from build123d import *

# Parameters (mm, degrees)
F0_R     = 4.4
F1_DEPTH = 1


with BuildPart() as f1:
    # F0 (on Front) → F1 (new body)
    with BuildSketch(Plane.XZ):
        with BuildLine():
            ThreePointArc((-1.4986815922, 5.1042757445), (-10.8737353251, 1.8109915545), (-1, 2.9275505456))
            ThreePointArc((-1, 2.9275505456), (-1.0654410934, 3.733855945), (-1.2600513589, 4.5190551417))
            ThreePointArc((-1.2600513589, 4.5190551417), (-1.3701106972, 4.81543959), (-1.4986815922, 5.1042757445))
        make_face()
        with Locations((-6, 2.9275505456)):
            Circle(F0_R, mode=Mode.SUBTRACT)
        with BuildLine():
            ThreePointArc((-1.4986815922, 5.1042757445), (-1.3701106972, 4.81543959), (-1.2600513589, 4.5190551417))
            add(Edge.make_bspline(
                [(-1.2600513589, 4.5190551417), (-0.3321453987, 5.1084347069), (0.2222434123, 5.0197322853), (1.305815297, 4.6493606322)],
                knots=[0, 0, 0, 0, 2.5691732555, 2.5691732555, 2.5691732555, 2.5691732555], degree=3))
            ThreePointArc((1.305815297, 4.6493606322), (1.408443121, 4.9068447194), (1.525181814, 5.1582459982))
            add(Edge.make_bspline(
                [(-1.4986815922, 5.1042757445), (0, 5.9878164902), (1.4394625627, 5.1295237069), (1.525181814, 5.1582459982)],
                knots=[0, 0, 0, 0, 0.9403135209, 0.9403135209, 0.9403135209, 0.9403135209], degree=3))
        make_face()
        with BuildLine():
            ThreePointArc((1.525181814, 5.1582459982), (1.408443121, 4.9068447194), (1.305815297, 4.6493606322))
            ThreePointArc((1.305815297, 4.6493606322), (5.1256212248, -1.9954019991), (11, 2.9275505456))
            ThreePointArc((11, 2.9275505456), (10.9952473554, 3.1455043436), (10.9809984568, 3.3630437989))
            ThreePointArc((10.9809984568, 3.3630437989), (10.9614239437, 3.5474476752), (10.9350249024, 3.7309988718))
            ThreePointArc((10.9350249024, 3.7309988718), (6.7558272917, 7.8700929182), (1.5306314581, 5.1691448079))
            add(Edge.make_bspline(
                [(1.525181814, 5.1582459982), (1.5306228506, 5.160069148), (1.5306095387, 5.165466158), (1.5306314581, 5.1691448079)],
                knots=[0.9403135209, 0.9403135209, 0.9403135209, 0.9403135209, 1, 1, 1, 1], degree=3))
        make_face()
        with Locations((6, 2.9275505456)):
            Circle(F0_R, mode=Mode.SUBTRACT)
        with BuildLine():
            ThreePointArc((10.9350249024, 3.7309988718), (10.9614239437, 3.5474476752), (10.9809984568, 3.3630437989))
            Line((10.9809984568, 3.3630437989), (11.1943203956, 3.3630437989))
            Line((11.1943203956, 3.3630437989), (11.1943203956, -15.5131826177))
            Line((11.1943203956, -15.5131826177), (11.5463633525, -15.5131826177))
            Line((11.5463633525, -15.5131826177), (11.5463633525, 3.7309988718))
            Line((11.5463633525, 3.7309988718), (10.9350249024, 3.7309988718))
        make_face()
    extrude(amount=F1_DEPTH)


solid = f1.part
Could you check a few things on this model? Use its own coordinates, in mm. A direction names the side the tool comes from. Give positions to 0.01 mm unless a question says otherwise; leave off trailing zeros. Loops run counter-clockwise (first coordinate to the right, second up) from the corner with the lowest first, then second, coordinate; pieces in that order, holes last. Notation, with made-up numbers: M 0.5,-17.75 L 55.5,-17.75 A15 cw 55.5,-0.75 Z; hole C 71,76.25 d7. An arc over 180 degrees is marked long. Answer as a JSON object with one key per item and string values.
Q1. Suppose I cut it at D-D, the plane y = -0.8. State how many separate pieces and enclosed holes the cut face has, plus the area to 3 significant figures.
Values found:
{"separate pieces": "1", "enclosed holes": "2", "area": "44.0 mm²"}
Q2. If I drill on probe 1 along X at (y, z) = (-0.25, 3); probe 2 along Z at (x, y) = (-6, -0.25); probe 3 along X at (y, z) = (-0.55, 6.5), over which ranges is the centre line in solid material (lowest first)? Write a range as [from, to].
Values found:
{"probe 1": "x = [-11, -10.4], [-1.6, -1], [1, 1.6], [10.4, 11], [11.19, 11.55]", "probe 2": "z = [-2.07, -1.47], [7.33, 7.93]", "probe 3": "x = [-9.5, -8.57], [-3.43, -2.5], [2.5, 3.43], [8.57, 9.5]"}
Q3. If we mould it in two halves opening along Z, with no side actions, what happens to faces 3 (the cylindrical face through (-10.396, -0.493, 3.121)), 4 (the cylindrical face through (6.843, -0.493, 7.856)), 5 (the flat face through (-1.4, -1, 3.2))? For each: pulls with the +Z half, pulls with the -Z half, needs draft (parallel to the pull), parting line crosses it, or undercut.
Values found:
{"face 3": "undercut", "face 4": "pulls with the +Z half", "face 5": "needs draft"}
Q4. For faces 1 (the flat face through (11.194, -0.5, -5.9)), 2 (the cylindrical face through (2.51, -0.49, 0.25)), which set-ups out of +Z, -Z, +X, -X, +Y, -Y let a thin tool reach every point of the face, with its end or its side?
Values found:
{"face 1": "-Z, +Y, -Y", "face 2": "+Y, -Y"}
Q5. Suppose I cut it at A-A, the plane x = -6. List the corners of the cut face in (y, z) for me, plus the area to 3 significant figures.
Values found:
{"outline": "M -1,-2.07 L 0,-2.07 L 0,-1.47 L -1,-1.47 Z; M -1,7.33 L 0,7.33 L 0,7.93 L -1,7.93 Z", "area": "1.20 mm²"}
Q6. Suppose I cut it at B-B, the plane z = -0.75. List the corners of the cut face in (x, y) for me.
Values found:
{"outline": "M -9.39,-1 L -8.42,-1 L -8.42,0 L -9.39,0 Z; M -3.58,-1 L -2.61,-1 L -2.61,0 L -3.58,0 Z; M 2.61,-1 L 3.58,-1 L 3.58,0 L 2.61,0 Z; M 8.42,-1 L 9.39,-1 L 9.39,0 L 8.42,0 Z; M 11.19,-1 L 11.55,-1 L 11.55,0 L 11.19,0 Z"}
Q7. Suppose I cut it at C-C, the plane x = -2.75. List the corners of the cut face in (y, z) for me.
Values found:
{"outline": "M -1,-0.87 L 0,-0.87 L 0,-0.04 L -1,-0.04 Z; M -1,5.89 L 0,5.89 L 0,6.73 L -1,6.73 Z"}
